Geometry check sheet. Reference: the model listing, model coordinates, mm. A direction names the side the tool comes from. Round coordinates to 2 decimals unless told otherwise and drop trailing zeros. Loops run counter-clockwise (first coordinate to the right, second up) from the corner with the lowest first, then second, coordinate; pieces in that order, holes last. Notation, with made-up numbers: (-20.5, 0) - (-10.5, 0) arc R19 ccw to (-10.5, 16) - close; hole circle Ø1 at (4.5, 17.25). An arc over 180 degrees is marked (long way). Answer as CSV lines item,"result". Start each with the question number.
1) Thickness scan on line 1 along Z through (x, y) = (-3, 2.75); line 2 along X through (y, z) = (6, -17); line 3 along Z through (x, y) = (5, 2). Record the ranges inside material, lowest first.
2) Draft check along Z on faces 1 (the flat face through (-3, -3, 66.5)), 2 (the cylindrical face through (-4.88, -1.08, -52.61)), 3 (the flat face through (0, 2, 78.5)). Enter one of: released by +Z, released by -Z, zero draft, split by the parting line, or undercut.
3) Access from +Z, -Z, +X, -X, +Y, -Y to the whole of each face (thin tool, end or side, straight path). Record for faces 4 (the cylindrical face through (0.33, -7.493, 0.588)), 5 (the cylindrical face through (-4.88, -1.08, 52.89)), 6 (the cylindrical face through (-4.88, -1.08, -72.42)), 7 (the cylindrical face through (-3.76, -0.83, 64.98)).
4) Cross-section at A-A on z = -65. Record the boundary of the cut face in (x, y).
5) Depth check by flat-ended pin: P1, Ø3, axis at y = -6, z = 55, coming from the +X side; P2, Ø4, axis at x = 2.5, z = 16, coming from the +Y side; P3, Ø1.5, axis at x = -3, z = 22.5, coming from the -Y side; P4, Ø1.3, axis at x = -2, y = -0.5, coming from the +Z side. Enter the tip coordinate at first touch or a pass-through.
6) Cross-section at B-B on z = 8. Record the boundary of the cut face in (x, y), and give its area (3 significant figures).
from build123d import *

# Parameters (mm, degrees)
ESQUISSE2_W             = 3
ESQUISSE2_H             = 3.85
CHANFREIN1_SIZE         = 0.5
ESQUISSE4_W             = 11.666620124
ESQUISSE4_H             = 1.663113932
ENL_V_MAT_EXTRU_2_DEPTH = 0.5


with BuildPart() as part:
    # Esquisse2 → Révolution1 (revolve)
    with BuildSketch(Plane(origin=(0, 0, 0), x_dir=(0, 0, -1), z_dir=(1, 0, 0))):
        Polygon((-78.5, 0), (-66.5, 0), (-66.5, 3.85), (-66.5, 5), (-78.5, 5), align=None)
        with Locations((-65, 1.925)):
            Rectangle(ESQUISSE2_W, ESQUISSE2_H)
        Polygon((-63.5, 3.85), (-63.5, 0), (-42.5, 0), (-42.5, 5), (-63.5, 5), align=None)
        Polygon((-42.5, 5), (-42.5, 0), (0, 0), (0, 7.5), (-42.5, 7.5), align=None)
        Polygon((0, 7.5), (0, 0), (42.5, 0), (42.5, 5), (42.5, 7.5), align=None)
        Polygon((42.5, 5), (42.5, 0), (63.5, 0), (63.5, 3.85), (63.5, 5), align=None)
        with Locations((65, 1.925)):
            Rectangle(ESQUISSE2_W, ESQUISSE2_H)
        Polygon((66.5, 3.85), (66.5, 0), (78.5, 0), (78.5, 5), (66.5, 5), align=None)
    revolve(axis=Axis((0, 0, 42.5), (0, 0, -1)))

    # Chanfrein1
    chanfrein1_edges = [part.edges().sort_by_distance(p)[0] for p in [
        (0, -5, 63.5),
        (0, -7.5, 42.5),
        (0, -7.5, -42.5),
        (0, -5, -63.5),
    ]]
    chamfer(chanfrein1_edges, length=CHANFREIN1_SIZE)

    # Esquisse4 → Enlèv. mat.-Extru.2 (cut)
    with BuildSketch(Plane(origin=(0, 0, -78.5), x_dir=(-1, 0, 0), z_dir=(0, 0, -1))):
        Rectangle(ESQUISSE4_W, ESQUISSE4_H)
    enl_v_mat_extru_2 = extrude(amount=-ENL_V_MAT_EXTRU_2_DEPTH, mode=Mode.SUBTRACT)

    # Symétrie2: Enlèv. mat.-Extru.2 across plane
    add(enl_v_mat_extru_2.mirror(Plane.XY), mode=Mode.SUBTRACT)


solid = part.part
Answer block:
1,line 1,"z = -78.5 to -66.5, -63.5 to 63.5, 66.5 to 78.5"
1,line 2,"x = -4.5 to 4.5"
1,line 3,"z = -42.5 to 42.5"
2,face 1,"undercut"
2,face 2,"zero draft"
2,face 3,"released by +Z"
3,face 4,"+Z, -Z"
3,face 5,"+Z"
3,face 6,"-Z"
3,face 7,"none"
4,outline,"circle Ø7.7 at (0, 0)"
5,P1,"stops at x = 2.18"
5,P2,"stops at y = 7.48"
5,P3,"stops at y = -7.15"
5,P4,"stops at z = 78.5"
6,outline,"circle Ø15 at (0, 0)"
6,area,"177 mm^2"
